The listing builds one solid part. Answer for the finished solid, in the listing's coordinates (mm). Coordinates: 2 decimals unless noted, no trailing zeros.
```python
from build123d import *

# Parameters (mm, degrees)
F0_W = 68.9707696438
F0_H = 71.5107694268
F4_T = -2.54


with BuildPart() as f3:
    # F0 (on Top) → F3 section 0
    with BuildSketch(Plane.XY):
        Rectangle(F0_W, F0_H)
    # F2 (on offset) → F3 section 1
    with BuildSketch(Plane.XY.offset(101.6)):
        Polygon((25.1069236547, 0), (0, 41.6169241071), (-40.9330762923, 0), (0, -36.7323085666), align=None)
    loft()

    # F4
    f4_openings = [f3.faces().sort_by_distance(p)[0] for p in [
        (-5.275384, 1.628205, 101.6),
    ]]
    offset(amount=F4_T, openings=f4_openings, kind=Kind.INTERSECTION)


solid = f3.part
```
1) Each of these flat-tipped pins is pushed along its axis until it touches: P1, Ø2, axis at x = -32.5, z = 47.5, coming from the -Y side; P2, Ø8, axis at x = 5, z = 18.5, coming from the -Y side; P3, Ø1.5, axis at x = -18.5, z = 73, coming from the -Y side. Where does it stop, or does it pass through?
2) Straight lines are drawn through the part: probe 1 along X at (y, z) = (21.5, 50); probe 2 along Y at (x, z) = (13.5, 10); probe 3 along X at (y, z) = (-32, 74.5). For each, find the intervals that lie inside material, in ascending order.
3) The mould has two halves that part along Z. Classify faces 1 (the flat face through (-1, 0, 2.54)), 2 (the flat face through (-1, 0, 0)), 3 (the flat face through (-18, 20, 101.6)): released by +Z, released by -Z, zero draft, split by the parting line, or undercut.
Working result:
1. P1: stops at y = -21
1. P2: stops at y = -34.04
1. P3: stops at y = -21.62
2. probe 1: x = -23.59 to -20.86, 15.6 to 22.14
2. probe 2: y = -34.89 to -32.34, 30.9 to 33.51
2. probe 3: x = 1.16 to 6.43, 8.14 to 10.99
3. face 1: undercut
3. face 2: released by -Z
3. face 3: released by +Z
